Geometry: final body of the model. Coordinates: model frame, mm. Face numbers are marked on the shaded views. A direction names the side the tool comes from. Round coordinates to 2 decimals unless told otherwise and drop trailing zeros. Write each loop counter-clockwise with the first axis right and the second up, starting at its lowest first coordinate (ties: lowest second). Pieces come first, ordered by that corner, then holes. Notation, with made-up numbers: M 61,74.5 L 86,74.5 A17 ccw 86,99.5 Z; hole C 44,8.25 d5. An arc over 180 degrees is marked long. Use one line per item in the form item = value. Start each with the question number.
Item 1: Reachability of the marked faces 4 and 5 from +Z, -Z, +X, -X, +Y, -Y: full face, straight path, thin tool, end or side. Return the list, or none.
Item 2: Pin query (flat end, axial travel): pin 1 Ø16 at (x, y) = (-9.5, -5) entering from -Z; pin 2 Ø5 at (x, y) = (2, -6) entering from -Z; pin 3 Ø3 at (y, z) = (-0.5, 48.5) entering from -X. Return the tip coordinate at first contact, or that it passes through.
Item 3: Pull-direction query (Y, two-part tool) for the marked faces 1, 2 and 3; classes: pulls with the +Y half, pulls with the -Y half, needs draft (parallel to the pull), parting line crosses it, or undercut.
Item 4: Section query D-D (y = -21.5). Return loops of the section in (x, z) (1 decimal).
Item 5: Ray query, probe 1 along X at (y, z) = (0, 17); probe 2 along X at (y, z) = (-8, 3.5); probe 3 along X at (y, z) = (0, 5) (1 decimal). Return the intervals inside material, ascending.
Item 6: Section query B-B (z = 59.5). State how many separate pieces and enclosed holes the cut face has, and give its area (3 significant figures).
Item 7: Section query C-C (x = -23). Return loops of the section in (y, z) (1 decimal).
from build123d import *

# Parameters (mm, degrees)
F0_R      = 17.4625
F0_R_2    = 1.8288
F0_R_3    = 7.9375
F1_DEPTH  = 38.1
F2_R      = 1.8288
F2_R_2    = 7.9375
F3_DEPTH  = 9.525
F4_R      = 1.8288
F5_DEPTH  = 17.4625
F6_R      = 9.525
F7_DEPTH  = 7.14375
F8_R      = 3.96875
F9_DEPTH  = 3.175
F10_SIZE  = 0.762
F11_SIZE2 = 1.27
F11_SIZE  = 1.27


with BuildPart() as f1:
    # F0 (on Top) → F1 (new body)
    with BuildSketch(Plane.XY):
        Circle(F0_R)
        with Locations((-9.5415221286, -9.5415221286)):
            Circle(F0_R_2, mode=Mode.SUBTRACT)
        Circle(F0_R_3, mode=Mode.SUBTRACT)
        with Locations((9.5415221286, 9.5415221286)):
            Circle(F0_R_2, mode=Mode.SUBTRACT)
    extrude(amount=F1_DEPTH)

    # F2 (on face) → F3 (join)
    with BuildSketch(Plane.XY.offset(38.1)):
        with BuildLine():
            Line((17.4625, -31.0967476626), (17.4625, 0))
            ThreePointArc((17.4625, 0), (-12.3478521665, -12.3478521665), (0, 17.4625))
            Line((0, 17.4625), (-31.0967476626, 17.4625))
            ThreePointArc((-31.0967476626, 17.4625), (-34.3477573384, 15.7701314818), (-34.8261527514, 12.1363575562))
            Line((-34.8261527514, 12.1363575562), (-26.851716639, -9.7732255955))
            ThreePointArc((-26.851716639, -9.7732255955), (-20.2055762724, -20.2055762724), (-9.7732255955, -26.851716639))
            Line((-9.7732255955, -26.851716639), (12.1363575562, -34.8261527514))
            ThreePointArc((12.1363575562, -34.8261527514), (15.7701314818, -34.3477573384), (17.4625, -31.0967476626))
        make_face()
        with Locations((13.49375, -31.0967476626)):
            Circle(F2_R, mode=Mode.SUBTRACT)
        with Locations((-31.0967476626, 13.49375)):
            Circle(F2_R, mode=Mode.SUBTRACT)
        with BuildLine():
            ThreePointArc((0, 17.4625), (-12.3478521665, -12.3478521665), (17.4625, 0))
            ThreePointArc((17.4625, 0), (12.3478521665, 12.3478521665), (0, 17.4625))
        make_face()
        with Locations((-9.5415221286, -9.5415221286)):
            Circle(F2_R, mode=Mode.SUBTRACT)
        Circle(F2_R_2, mode=Mode.SUBTRACT)
        with Locations((9.5415221286, 9.5415221286)):
            Circle(F2_R, mode=Mode.SUBTRACT)
    extrude(amount=F3_DEPTH)

    # F4 (on face) → F5 (join)
    with BuildSketch(Plane.XY.offset(47.625)):
        with BuildLine():
            Line((-34.8261527514, 12.1363575562), (-26.851716639, -9.7732255955))
            ThreePointArc((-26.851716639, -9.7732255955), (-20.2055762724, -20.2055762724), (-9.7732255955, -26.851716639))
            Line((-9.7732255955, -26.851716639), (12.1363575562, -34.8261527514))
            ThreePointArc((12.1363575562, -34.8261527514), (17.2231550887, -32.4541401064), (14.8511424438, -27.3673425739))
            Line((14.8511424438, -27.3673425739), (-7.0584407079, -19.3929064615))
            ThreePointArc((-7.0584407079, -19.3929064615), (-14.5929161967, -14.5929161967), (-19.3929064615, -7.0584407079))
            Line((-19.3929064615, -7.0584407079), (-27.3673425739, 14.8511424438))
            ThreePointArc((-27.3673425739, 14.8511424438), (-32.4541401064, 17.2231550887), (-34.8261527514, 12.1363575562))
        make_face()
        with Locations((13.49375, -31.0967476626)):
            Circle(F4_R, mode=Mode.SUBTRACT)
        with Locations((-31.0967476626, 13.49375)):
            Circle(F4_R, mode=Mode.SUBTRACT)
    extrude(amount=F5_DEPTH)

    # F6 (on face) → F7 (cut)
    with BuildSketch(Plane(origin=(0, 0, 0), x_dir=(1, 0, 0), z_dir=(0, 0, -1))):
        Circle(F6_R)
    extrude(amount=-F7_DEPTH, mode=Mode.SUBTRACT)

    # F8 (on face) → F9 (join)
    with BuildSketch(Plane(origin=(0, 0, 0), x_dir=(1, 0, 0), z_dir=(0, 0, -1))):
        with Locations((-9.5415221286, -9.5415221286)):
            Circle(F8_R)
        with Locations((9.5415221286, 9.5415221286)):
            Circle(F8_R)
    extrude(amount=F9_DEPTH)

    # F10
    f10_edges = [f1.edges().sort_by_distance(p)[0] for p in [
        (5.572772, -9.541522, -3.175),
        (-13.510272, 9.541522, -3.175),
    ]]
    chamfer(f10_edges, length=F10_SIZE)

    # F11
    f11_edges = [f1.edges().sort_by_distance(p)[0] for p in [
        (7.712722, 9.541522, 47.625),
        (-11.370322, -9.541522, 47.625),
    ]]
    chamfer(f11_edges, length=F11_SIZE, length2=F11_SIZE2)


solid = f1.part
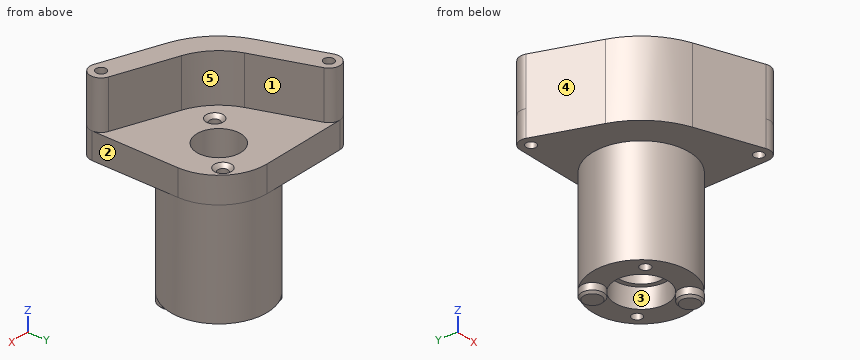
Working result:
q1.face_4 = +Z, -Z, -X, -Y
q1.face_5 = +Z, +X, +Y
q2.pin_1 = 0
q2.pin_2 = 7.14
q2.pin_3 = -30.77
q3.face_1 = pulls with the +Y half
q3.face_2 = needs draft
q3.face_3 = undercut
q4.outline = M -18.8,38.1 L 17.5,38.1 L 17.5,47.6 L -1.3,47.6 L -1.3,65.1 L -18.8,65.1 Z
q5.probe_1 = -17.46 to -7.94, 7.94 to 17.46
q5.probe_2 = -15.52 to -10.53, -8.56 to -5.17, 5.17 to 15.52
q5.probe_3 = -17.5 to -9.5, 9.5 to 17.5
q6.separate_pieces = 1
q6.enclosed_holes = 2
q6.area = 569 mm²
q7.outline = M -17,38.1 L 17.5,38.1 L 17.5,47.6 L 2.9,47.6 L 2.9,65.1 L -17,65.1 Z
